The drawing under review shows one solid part. Ordinate dimensions are in mm from its lowest x, y, z. A direction names the side the tool comes from. Give positions to 0.01 mm unless a question says otherwise; leave off trailing zeros. Order: outer loops, then holes, each group sorted by start corner. A loop starts at its lowest first (then second) coordinate and runs counter-clockwise, first axis right, second up. Notation, with made-up numbers: (62, 15) - (100, 15) arc R9 cw to (100, 25) - close; hole circle Ø11 at (41.25, -5.5). An arc over 180 degrees is marked (long way). Answer as a JSON object with one key per item and string values. Group by question number.
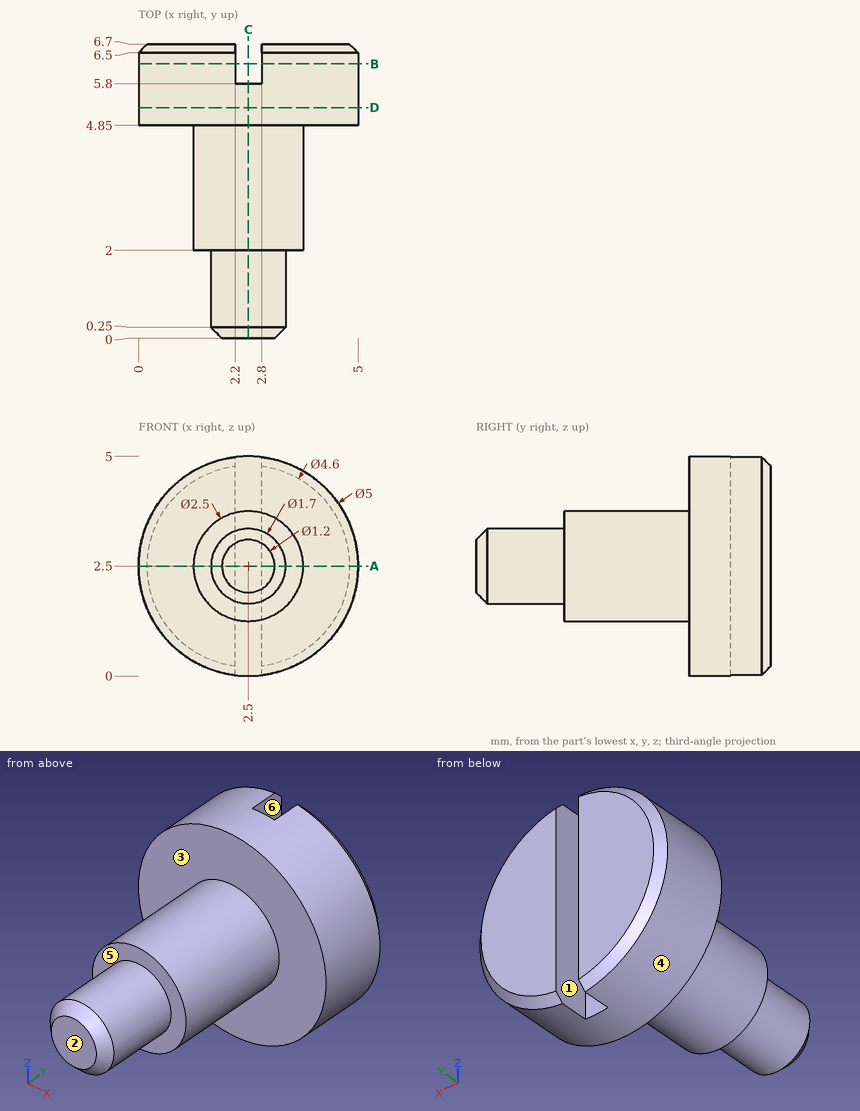
1) Consider section C-C (x = 2.5). Give the boundary of the cut face in (y, z), plus the area to 3 significant figures.
2) For pin 1 (3 mm diameter, centred on x = 3, z = 2.5, fed in from -Y); pin 2 (2 mm diameter, centred on y = 1, z = 4.5, fed in from -X); pin 3 (3 mm diameter, centred on x = 1, y = 3, fed in from -Z); pin 4 (0.7 mm diameter, centred on y = 6.5, z = 2, fed in from +X), all flat-tipped, find the tip position at first contact; note any pin that passes through.
3) Consider section A-A (z = 2.5). Give the boundary of the cut face in (x, y), plus the area to 3 significant figures.
4) For line 1 (X direction, y = 6.25, z = 1.75); line 2 (Y direction, x = 0.65, z = 1.8); line 3 (Y direction, x = 2.45, z = 1.2), list the stretches that pass through material, from the lowest coordinate up.
5) Mouldability with a two-part tool opening along X and no side actions: class the marked faces 4, 5 and 6 as released by +X, released by -X, zero draft, split by the parting line, or undercut.
6) Consider section B-B (y = 6.25). Give the boundary of the cut face in (x, z).
7) Consider section D-D (y = 5.25). Give the boundary of the cut face in (x, z), plus the area to 3 significant figures.
8) For the marked faces 1, 2 and 3, list the 3-axis set-ups (+Z, -Z, +X, -X, +Y, -Y) from which the entire face can be reached by the end or side of a thin tool; tool diameter is ignored.
Result set:
{
 "1": {"outline": "(0, 1.9) - (0.25, 1.65) - (2, 1.65) - (2, 1.25) - (4.85, 1.25) - (4.85, 0) - (5.8, 0) - (5.8, 5) - (4.85, 5) - (4.85, 3.75) - (2, 3.75) - (2, 3.35) - (0.25, 3.35) - (0, 3.1) - close", "area": "15.2 mm2"},
 "2": {"pin 1": "stops at y = 0", "pin 2": "passes through", "pin 3": "stops at z = 1.25", "pin 4": "stops at x = 5"},
 "3": {"outline": "(0, 4.85) - (1.25, 4.85) - (1.25, 2) - (1.65, 2) - (1.65, 0.25) - (1.9, 0) - (3.1, 0) - (3.35, 0.25) - (3.35, 2) - (3.75, 2) - (3.75, 4.85) - (5, 4.85) - (5, 6.5) - (4.8, 6.7) - (2.8, 6.7) - (2.8, 5.8) - (2.2, 5.8) - (2.2, 6.7) - (0.2, 6.7) - (0, 6.5) - close", "area": "19.1 mm2"},
 "4": {"line 1": "x = 0.12 to 2.2, 2.8 to 4.88", "line 2": "y = 4.85 to 6.7", "line 3": "y = 4.85 to 5.8"},
 "5": {"face 4": "split by the parting line", "face 5": "zero draft", "face 6": "undercut"},
 "6": {"outline": "(2.2, 0.02) - (2.2, 4.98) arc R2.5 ccw to start; (2.8, 0.02) arc R2.5 ccw to (2.8, 4.98) - close"},
 "7": {"outline": "circle Ø5 at (2.5, 2.5)", "area": "19.6 mm2"},
 "8": {"face 1": "+Z, -Z, +Y", "face 2": "+Z, -Z, +X, -X, -Y", "face 3": "-Y"}
}
